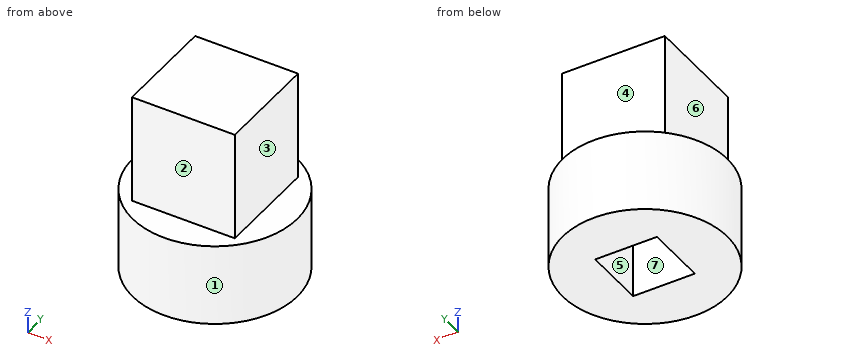
```python
from build123d import *

# Parameters (mm, degrees)
SKETCH079_W     = 3.75
SKETCH079_H     = 3.75
PAD046_DEPTH    = 4
SKETCH080_R     = 3
PAD047_DEPTH    = 3
SKETCH081_W     = 2.25
SKETCH081_H     = 2.25
POCKET034_DEPTH = 3


with BuildPart() as part:
    # Sketch079 → Pad046 (new body)
    with BuildSketch(Plane(origin=(0, 0, 22), x_dir=(1, 0, 0), z_dir=(0, 0, -1))):
        with Locations((5.5, 22.5)):
            Rectangle(SKETCH079_W, SKETCH079_H)
    extrude(amount=-PAD046_DEPTH)

    # Sketch080 (on Face5 of Pad046) → Pad047 (join)
    with BuildSketch(Plane(origin=(0, 0, 22), x_dir=(1, 0, 0), z_dir=(0, 0, -1))):
        with Locations((5.5, 22.5)):
            Circle(SKETCH080_R)
    extrude(amount=PAD047_DEPTH)

    # Sketch081 (on Face3 of Pad047) → Pocket034 (cut)
    with BuildSketch(Plane(origin=(0, 0, 19), x_dir=(1, 0, 0), z_dir=(0, 0, -1))):
        with Locations((5.5, 22.5)):
            Rectangle(SKETCH081_W, SKETCH081_H)
    extrude(amount=-POCKET034_DEPTH, mode=Mode.SUBTRACT)


solid = part.part
```
CAD build for the part. Positions are in the model's coordinates, mm. Face numbers are marked on the shaded views. A direction names the side the tool comes from. Give positions to 0.01 mm unless a question says otherwise; leave off trailing zeros. Order: outer loops, then holes, each group sorted by start corner. A loop starts at its lowest first (then second) coordinate and runs counter-clockwise, first axis right, second up. Notation, with made-up numbers: M 61,14 L 119,14 A32 ccw 119,53 Z; hole C -5,39 d1. An arc over 180 degrees is marked long. Put each result on its own line as item: value. Start each with the question number.
(1) Flat gauge pins, fed straight in: pin 1 Ø1.9 at (y, z) = (-22.5, 24) entering from -X (3 decimals); pin 2 Ø1.1 at (x, z) = (5, 23) entering from +Y (3 decimals); pin 3 Ø0.7 at (x, y) = (5.5, -23) entering from -Z. Where does each tip first touch, or does it go through?
(2) Saw through at C-C, the plane x = 5.5. Write the cut outline in (y, z) (3 decimals), then the cut area to 4 significant figures.
(3) Mould opens along X. For the marked faces 4, 5, 6 and 7 say: +X half, -X half, draft (parallel to the pull), parting line (faces both ways), or undercut.
(4) Saw through at A-A, the plane y = -22.5. Write the cut outline in (x, z) (3 decimals), then the cut area to 4 significant figures.
(5) Saw through at D-D, the plane z = 23.25. Write the cut outline in (x, y) (3 decimals).
(6) Saw through at B-B, the plane z = 21.25. Write the cut outline in (x, y) (3 decimals).
(7) Which spindle directions (+Z, -Z, +X, -X, +Y, -Y) get a long thin tool onto all of the face, cutting with end or side? Do the marked faces 1, 2 and 3. Say none if no direction does.
(8) Drill centre lines: line 1 along X through (y, z) = (-22.4, 20.75) (3 decimals); line 2 along Z through (x, y) = (5.25, -22); line 3 along Y through (x, z) = (6.15, 21.25) (3 decimals). Where is each one in solid material? Low to high.
Check result:
1. pin 1: stops at x = 3.625
1. pin 2: stops at y = -20.625
1. pin 3: stops at z = 22
2. outline: M -25.5,19 L -23.625,19 L -23.625,22 L -21.375,22 L -21.375,19 L -19.5,19 L -19.5,22 L -20.625,22 L -20.625,26 L -24.375,26 L -24.375,22 L -25.5,22 Z
2. area: 26.25 mm2
3. face 4: draft
3. face 5: undercut
3. face 6: -X half
3. face 7: undercut
4. outline: M 2.5,19 L 4.375,19 L 4.375,22 L 6.625,22 L 6.625,19 L 8.5,19 L 8.5,22 L 7.375,22 L 7.375,26 L 3.625,26 L 3.625,22 L 2.5,22 Z
4. area: 26.25 mm2
5. outline: M 3.625,-24.375 L 7.375,-24.375 L 7.375,-20.625 L 3.625,-20.625 Z
6. outline: C 5.5,-22.5 d6; hole M 4.375,-23.625 L 6.625,-23.625 L 6.625,-21.375 L 4.375,-21.375 Z
7. face 1: +Z, -Z
7. face 2: +Z, +X, -X, -Y
7. face 3: +Z, +X, +Y, -Y
8. line 1: x = 2.502 to 4.375, 6.625 to 8.498
8. line 2: z = 22 to 26
8. line 3: y = -25.429 to -23.625, -21.375 to -19.571
